Autodesk Inventor part; units mm, degrees
ref_plane "Work Plane1" through (0, 5, 0) normal (0, 1, 0) x (-1, 0, 0)
ref_plane "Work Plane2" through (0, 36, 0) normal (0, 1, 0) x (-1, 0, 0)
ref_plane "YZ Plane" through (0, 0, 0) normal (1, 0, 0) x (0, 1, 0)
sketch "Sketch1" plane through (0, 0, 0) normal (1, 0, 0) x (0, 1, 0)
  line L0 (27, 0) -> (0, 0)
  line L1 (27, 0) -> (31.5, -4.5)
  line L2 (31.5, -4.5) -> (31.5, -5.5)
  line L3 (27, 0) -> (27, -13.1503) construction
  line L4 (31.5, -5.5) -> (30.5, -5.5)
  line L5 (30.5, -5.5) -> (30.5, -6.5)
  line L6 (30.5, -6.5) -> (31.5, -6.5)
  line L7 (31.5, -6.5) -> (31.5, -84)
  line L8 (31.5, -84) -> (0, -84)
  line L9 (0, -84) -> (0, 0)
  dimension "d0" = 27
  dimension "d1" = 31.5
  dimension "d2" = 45
  dimension "d5" = 1
  dimension "d6" = 1
  dimension "d7" = 1
  dimension "d8" = 1
  dimension "d9" = 84
revolve "Revolution1" add sketch "Sketch1" angle 360 about axis through (0, 0, -84) along (0, 0, 1)
sketch "Sketch2" plane through (0, 0, 0) normal (0, 0, 1) x (1, 0, 0)
  circle A0 centre (-15.5563, 15.5563) radius 2
  line L0 (-15.5563, 15.5563) -> (0, 0) construction
  line L1 (0, 0) -> (-12.1027, 0) construction
  circle A1 centre (-15.5563, -15.5563) radius 2
  circle A2 centre (15.5563, -15.5563) radius 2
  circle A3 centre (15.5563, 15.5563) radius 2
  dimension "d11" = 4
  dimension "d12" = 22
  dimension "d13" = 45
  dimension "d16" = 360
extrude "Extrusion1" cut sketch "Sketch2" against normal blind 5
thread "Thread1"
thread "Thread2"
thread "Thread3"
thread "Thread4"
sketch "Sketch3" plane through (0, 0, 0) normal (0, 0, 1) x (1, 0, 0)
  circle A0 centre (0, 0) radius 5
  dimension "d28" = 10
extrude "Extrusion2" add sketch "Sketch3" along normal blind 30
chamfer "Chamfer1" distance 0.5 angle 45 1 edges at (-5, 0, 30)
ref_plane "Work Plane1" through (0, 5, 0) normal (0, 1, 0) x (-1, 0, 0)
sketch "Sketch4" plane through (0, 5, 0) normal (0, 1, 0) x (-1, 0, 0)
  line L0 (0, 13) -> (0, 24) construction
  line L1 (1.5, 13) -> (1.5, 24)
  line L2 (-1.5, 24) -> (-1.5, 13)
  arc A0 (-1.5, 13) -> (1.5, 13) centre (0, 13) ccw
  arc A1 (1.5, 24) -> (-1.5, 24) centre (0, 24) ccw
  line L3 (5, 29.5) -> (-5, 29.5) construction
  point P0 (0, 0)
  point P1 (0, 18.5)
  point P2 (0, 29.5)
  point P3 (0, 25.5)
  dimension "d35" = 11
  dimension "d36" = 3
  dimension "d37" = 4
extrude "Extrusion3" cut sketch "Sketch4" against normal blind 1.5
ref_plane "Work Plane2" through (0, 36, 0) normal (0, 1, 0) x (-1, 0, 0)
sketch "Sketch5" plane through (0, 36, 0) normal (0, 1, 0) x (-1, 0, 0)
  line L0 (14.1999, -66.6752) -> (-12.4029, -66.6752) construction
  line L1 (-12.4029, -66.6752) -> (-12.4029, -14.1495) construction
  line L2 (-12.4029, -14.1495) -> (14.1999, -14.1495) construction
  line L3 (14.1999, -14.1495) -> (14.1999, -66.6752) construction
  point P0 (0, 0)
decal "Decal1"
sketch "Sketch6" plane through (0, 0, -84) normal (0, 0, -1) x (-1, 0, 0)
  circle A0 centre (0, 0) radius 31.5
  circle A1 centre (0, 0) radius 31
  dimension "d52" = 0.5
extrude "Extrusion4" cut sketch "Sketch6" against normal blind 14
chamfer "Chamfer2" distance 0.5 angle 45 1 edges at (31, 0, -70)
sketch "Sketch7" plane through (0, 0, 0) normal (0, 0, 1) x (1, 0, 0)
  circle A0 centre (0, 0) radius 11
  dimension "d58" = 22
extrude "Extrusion5" cut sketch "Sketch7" against normal blind 3
sketch "Sketch8" plane through (0, 0, -3) normal (0, 0, 1) x (1, 0, 0)
  circle A0 centre (0, 0) radius 7
  dimension "d61" = 14
extrude "Extrusion6" add sketch "Sketch8" along normal blind 4
sketch "Sketch9" plane through (0, 0, -3) normal (0, 0, 1) x (1, 0, 0)
  circle A0 centre (0, 0) radius 11
  circle A1 centre (0, 0) radius 10.5
  circle A2 centre (0, 0) radius 9.8
  circle A3 centre (0, 0) radius 8.8
  circle A4 centre (0, 0) radius 8.4
  circle A5 centre (0, 0) radius 7.65
  circle A6 centre (0, 0) radius 7
  dimension "d64" = 0.5
  dimension "d65" = 0.7
  dimension "d66" = 1
  dimension "d69" = 0.4
  dimension "d70" = 0.75
extrude "Extrusion7" cut sketch "Sketch9" against normal blind 0.5 contours A1
extrude "Extrusion8" cut sketch "Sketch9" against normal blind 0.5 contours A3
fillet "Fillet1" radius 0.35 2 edges at (-9.8, 0, -3) (-8.8, 0, -3)
extrude "Extrusion9" cut sketch "Sketch9" against normal blind 0.5 contours A5
properties part number "Flipsky E-Board Motor 6384 190KV"
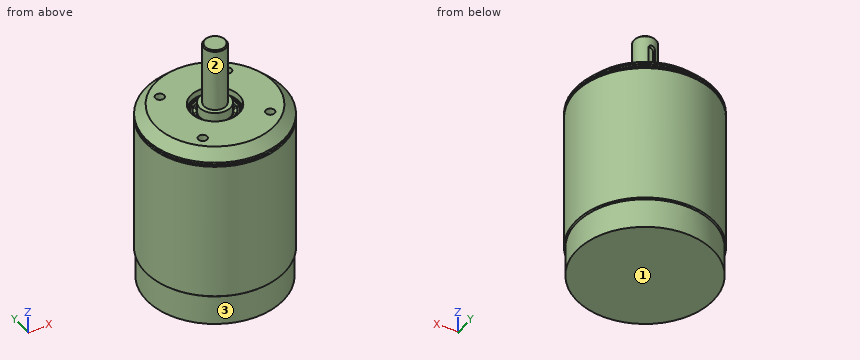
Work out the finished part from the listing and answer in its coordinate system (mm). Face numbers are marked on the shaded views. A direction names the side the tool comes from. Round coordinates to 2 decimals unless told otherwise and drop trailing zeros. Loops run counter-clockwise (first coordinate to the right, second up) from the corner with the lowest first, then second, coordinate; pieces in that order, holes last. Notation, with made-up numbers: (-19.75, 85.25) -> (19.25, 85.25) arc R24 cw to (19.25, 117.25) -> close; hole circle Ø5 at (14, 89). An arc over 180 degrees is marked (long way). Use one line per item in the form item = value.
(1) Flat-ended cylindrical pins translate along their axes: P1, Ø4, axis at x = -7.5, z = -24.5, coming from the +Y side; P2, Ø5, axis at x = -13, z = -2, coming from the +Y side; P3, Ø1.2, axis at x = 15.5, y = 15.5, coming from the +Z side. Find the tip coordinate at first contact, or state that the pin passes through.
Answer list:
P1 = 31.02
P2 = 28.9
P3 = -5
(2) Find section A-A on z = -15. Give the vertices of the cut face in (x, y).
Answer list:
outline = circle Ø63 at (0, 0)
(3) Straight lines are drawn through the part: line 1 (Z direction, x = 11, y = -2); line 2 (X direction, y = 5.5, z = -37); line 3 (Y direction, x = -6.5, z = -56.5). For each, find the intervals that lie inside material, in ascending order.
Answer list:
line_1 = -84 to 0
line_2 = -31.02 to 31.02
line_3 = -30.82 to 30.82
(4) A tool of negligible diameter and unlimited length cuts with its end or side. For the marked faces 1, 2 and 3, from which of +Z, -Z, +X, -X, +Y, -Y can it reach the whole face along a straight path? Write none if from no direction.
Answer list:
face_1 = -Z, +X, -X, +Y, -Y
face_2 = +Z
face_3 = -Z
